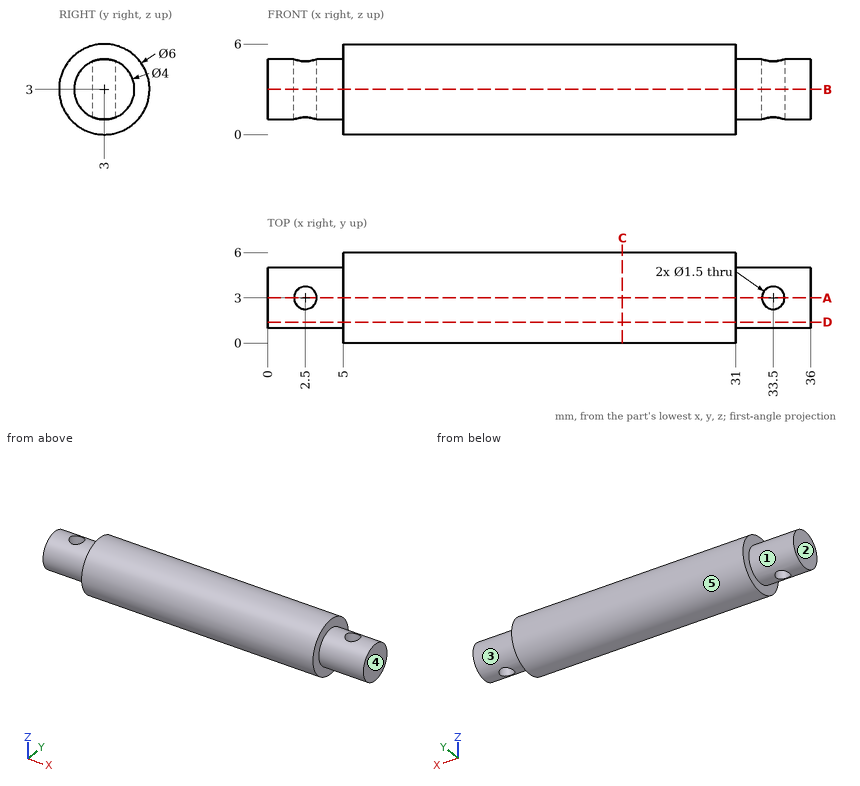
Input: dimensioned drawing with shaded views. Units: mm. Origin: part minimum x, y, z. A direction names the side the tool comes from. Coordinates: 2 decimals unless noted, no trailing zeros. Write each loop counter-clockwise with the first axis right and the second up, starting at its lowest first coordinate (ties: lowest second). Pieces come first, ordered by that corner, then holes. Notation, with made-up numbers: M 15,71.25 L 28,71.25 A17 ccw 28,86.25 Z; hole C -6,0 d6. An arc over 180 degrees is marked long. Use one line per item in the form item = value.
Q1. Material intervals for probe 1 along X at (y, z) = (3.05, 3.15); probe 2 along Y at (x, z) = (2.5, 3.1); probe 3 along X at (y, z) = (3.2, 0.4), sorted ascending. Write a range as from..to.
Answer below:
probe_1 = 0..1.75, 3.25..32.75, 34.25..36
probe_2 = 1..2.25, 3.75..5
probe_3 = 5..31
Q2. Section D-D (y = 1.4). Return loops of the section in (x, z).
Answer below:
outline = M 0,1.8 L 5,1.8 L 5,0.46 L 31,0.46 L 31,1.8 L 36,1.8 L 36,4.2 L 31,4.2 L 31,5.54 L 5,5.54 L 5,4.2 L 0,4.2 Z
Q3. Section B-B (z = 3). Return loops of the section in (x, y).
Answer below:
outline = M 0,1 L 5,1 L 5,0 L 31,0 L 31,1 L 36,1 L 36,5 L 31,5 L 31,6 L 5,6 L 5,5 L 0,5 Z; hole C 2.5,3 d1.5; hole C 33.5,3 d1.5
Q4. First-contact query: pin 1 (1.5 mm diameter, centred on x = 28.5, z = 2, fed in from +Y); pin 2 (1 mm diameter, centred on y = 0.5, z = 2.5, fed in from +X); pin 3 (2.5 mm diameter, centred on x = 2.5, y = 3, fed in from -Z). Flat tips, straight axial feed; report the tip coordinate or a pass-through.
Answer below:
pin_1 = 5.99
pin_2 = 31
pin_3 = 1
Q5. Section A-A (y = 3). Return loops of the section in (x, z).
Answer below:
outline = M 0,1 L 1.75,1 L 1.75,5 L 0,5 Z; M 3.25,1 L 5,1 L 5,0 L 31,0 L 31,1 L 32.75,1 L 32.75,5 L 31,5 L 31,6 L 5,6 L 5,5 L 3.25,5 Z; M 34.25,1 L 36,1 L 36,5 L 34.25,5 Z
Q6. Set-up query: the marked faces 1, 2 and 3. Return all of +Z, -Z, +X, -X, +Y, -Y with unobstructed straight access to the full face (end or side cutting, diameter ignored); none if empty.
Answer below:
face_1 = -X
face_2 = +Z, -Z, -X, +Y, -Y
face_3 = +X
Q7. Section C-C (x = 23.5). Return loops of the section in (y, z), plus the area to 3 significant figures.
Answer below:
outline = C 3,3 d6
area = 28.3 mm²
Q8. Draft query along Z for the marked faces 4 and 5. Return one class per face: released by +Z, released by -Z, zero draft, split by the parting line, or undercut.
Answer below:
face_4 = zero draft
face_5 = split by the parting line
